Design review of the part shown in the three views and the two pictorial views. Dimensions are in mm from the part's minimum x, y and z. A direction names the side the tool comes from. Coordinates: 2 decimals unless noted, no trailing zeros. Loops run counter-clockwise (first coordinate to the right, second up) from the corner with the lowest first, then second, coordinate; pieces in that order, holes last.
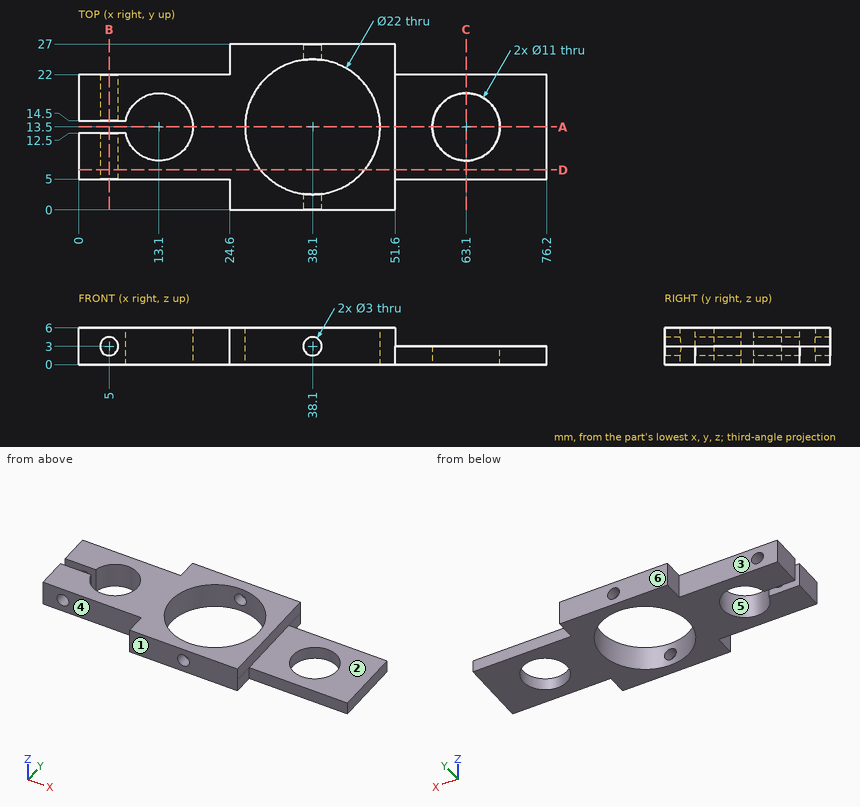
Q1. Machinability: for the marked faces 1, 2, 3 and 4, which of the approach directions +Z, -Z, +X, -X, +Y, -Y give a long, thin tool a straight path to every point of the face, cutting with its end or side? Answer none if there is none.
Q2. For pin 1 Ø1 at (y, z) = (24, 3.5) entering from -X; pin 2 Ø2.5 at (x, z) = (5, 3) entering from +Y; pin 3 Ø0.9 at (y, z) = (25, 2) entering from +X; pin 4 Ø1.5 at (x, y) = (63.5, 4.5) entering from +Z, all flat-tipped, find the tip position at first contact; note any pin that passes through.
Q3. Consider section A-A (y = 13.5). State the section outline as (x, z) points.
Q4. Wall thickness on probe 1 along Z at (x, y) = (38.1, 26.1); probe 2 along X at (y, z) = (20.25, 2.25); probe 3 along X at (y, z) = (13, 0.5): over which ranges is each line inside the solid? List them lowest first.
Q5. The part is to be moulded in two halves that separate along X. For the marked faces 5 and 6, say which applies: +X half, -X half, draft (parallel to the pull), parting line (faces both ways), or undercut.
Q6. Consider section B-B (x = 5). State the section outline as (y, z) points, then the cut area to 3 significant figures.
Q7. Consider section C-C (x = 63.1). State the section outline as (y, z) points.
Q8. Consider section D-D (y = 6.5). State the section outline as (x, z) points.
Model answer:
1. face 1: +Z, -Z, +X, -X, -Y
1. face 2: +Z, +X, +Y, -Y
1. face 3: +Z, -Z, -X, +Y
1. face 4: +Z, -Z, -X, -Y
2. pin 1: stops at x = 24.6
2. pin 2: passes through
2. pin 3: stops at x = 51.6
2. pin 4: stops at z = 3
3. outline: (18.6, 0) - (27.1, 0) - (27.1, 6) - (18.6, 6) - close; (49.1, 0) - (57.6, 0) - (57.6, 3) - (51.6, 3) - (51.6, 6) - (49.1, 6) - close; (68.6, 0) - (76.2, 0) - (76.2, 3) - (68.6, 3) - close
4. probe 1: z = 0 to 1.5, 4.5 to 6
4. probe 2: x = 0 to 3.7, 6.3 to 29.41, 46.79 to 76.2
4. probe 3: x = 18.58 to 27.11, 49.09 to 57.62, 68.58 to 76.2
5. face 5: undercut
5. face 6: draft
6. outline: (5, 0) - (12.5, 0) - (12.5, 1.5) - (5, 1.5) - close; (5, 4.5) - (12.5, 4.5) - (12.5, 6) - (5, 6) - close; (14.5, 0) - (22, 0) - (22, 1.5) - (14.5, 1.5) - close; (14.5, 4.5) - (22, 4.5) - (22, 6) - (14.5, 6) - close
6. area: 45.0 mm2
7. outline: (5, 0) - (8, 0) - (8, 3) - (5, 3) - close; (19, 0) - (22, 0) - (22, 3) - (19, 3) - close
8. outline: (0, 0) - (29.61, 0) - (29.61, 6) - (0, 6) - close; (46.59, 0) - (76.2, 0) - (76.2, 3) - (51.6, 3) - (51.6, 6) - (46.59, 6) - close; hole circle Ø3 at (5, 3)
